Work out the finished part from the listing and answer in its coordinate system (mm). A direction names the side the tool comes from. Coordinates: 2 decimals unless noted, no trailing zeros. Loops run counter-clockwise (first coordinate to the right, second up) from the corner with the lowest first, then second, coordinate; pieces in that order, holes last. Notation, with made-up numbers: (-26.75, 59.25) -> (23.25, 59.25) arc R24 ccw to (23.25, 92.25) -> close; hole circle Ø5 at (1.5, -27). An arc over 180 degrees is marked (long way). Use a Markdown table: item, result.
from build123d import *

# Parameters (mm, degrees)
CYLINDER004_R     = 2.5
CYLINDER004_DEPTH = 16.6
CYLINDER005_R     = 1.5
CYLINDER005_DEPTH = 9
CYLINDER008_R     = 1.5
CYLINDER008_DEPTH = 9
CYLINDER007_R     = 4.8
CYLINDER007_DEPTH = 7.3
CHAMFER003_SIZE   = 0.2
CYLINDER002_R     = 9
CYLINDER002_DEPTH = 0.7
CHAMFER_SIZE      = 0.2
CYLINDER003_R     = 9
CYLINDER003_DEPTH = 0.7
CHAMFER001_SIZE   = 0.2
CYLINDER_R        = 0.6
CYLINDER_DEPTH    = 7.6
ARRAY_COUNT       = 20
CYLINDER001_R     = 6.7
CYLINDER001_DEPTH = 7.6


with BuildPart() as cilindro004:
    # Cylinder004 → Cylinder004 (new body)
    with BuildSketch(Plane.XY):
        Circle(CYLINDER004_R)
    extrude(amount=CYLINDER004_DEPTH)


with BuildPart() as cilindro005:
    # Cylinder005 → Cylinder005 (new body)
    with BuildSketch(Plane(origin=(1, 0, 3.5), x_dir=(0, 0, -1), z_dir=(1, 0, 0))):
        Circle(CYLINDER005_R)
    extrude(amount=CYLINDER005_DEPTH)


with BuildPart() as fusion001:
    # Cylinder008 → Cylinder008 (new body)
    with BuildSketch(Plane(origin=(0, -1, 3.5), x_dir=(0, 0, -1), z_dir=(0, -1, 0))):
        Circle(CYLINDER008_R)
    extrude(amount=CYLINDER008_DEPTH)

    # Fusion001: union Cilindro005
    add(cilindro005.part)


with BuildPart() as cut001:
    # Cylinder007 → Cylinder007 (new body)
    with BuildSketch(Plane.XY):
        Circle(CYLINDER007_R)
    extrude(amount=CYLINDER007_DEPTH)

    # Chamfer003
    chamfer003_edges = [cut001.edges().sort_by_distance(p)[0] for p in [
        (-4.8, 0, 7.3),
    ]]
    chamfer(chamfer003_edges, length=CHAMFER003_SIZE)

    # Cut001: cut Fusion001
    add(fusion001.part, mode=Mode.SUBTRACT)


with BuildPart() as cut001_1:
    # Cut001 placement: moved
    add(cut001.part.moved(Location((0, 0, 9))))


with BuildPart() as chamfer_body:
    # Cylinder002 → Cylinder002 (new body)
    with BuildSketch(Plane.XY):
        Circle(CYLINDER002_R)
    extrude(amount=CYLINDER002_DEPTH)

    # Chamfer
    chamfer_edges = [chamfer_body.edges().sort_by_distance(p)[0] for p in [
        (-9, 0, 0.7),
    ]]
    chamfer(chamfer_edges, length=CHAMFER_SIZE)


with BuildPart() as chamfer001:
    # Cylinder003 → Cylinder003 (new body)
    with BuildSketch(Plane.XY.offset(8.3)):
        Circle(CYLINDER003_R)
    extrude(amount=CYLINDER003_DEPTH)

    # Chamfer001
    chamfer001_edges = [chamfer001.edges().sort_by_distance(p)[0] for p in [
        (-9, 0, 8.3),
    ]]
    chamfer(chamfer001_edges, length=CHAMFER001_SIZE)


with BuildPart() as array:
    # Cylinder → Cylinder (new body)
    with BuildSketch(Plane(origin=(6.7, 0, 0), x_dir=(1, 0, 0), z_dir=(0, 0, 1))):
        Circle(CYLINDER_R)
    extrude(amount=CYLINDER_DEPTH)

    # Array: Array ×20 about axis
    array_axis = Axis((0, 0, 0), (0, 0, 1))


with BuildPart() as array_1:
    add(array.part)
    for i in range(1, ARRAY_COUNT):
        add(array.part.rotate(array_axis, i * 360 / ARRAY_COUNT))


with BuildPart() as obj1:
    # Cylinder001 → Cylinder001 (new body)
    with BuildSketch(Plane.XY):
        Circle(CYLINDER001_R)
    extrude(amount=CYLINDER001_DEPTH)

    # Cut: cut Array
    add(array_1.part, mode=Mode.SUBTRACT)


with BuildPart() as obj1_1:
    # Cut placement: moved
    add(obj1.part.moved(Location((0, 0, 0.7))))

    # Fusion: union Chamfer body, Chamfer001
    add(chamfer_body.part)
    add(chamfer001.part)

    # Fusion002: union Cut001
    add(cut001_1.part)

    # Cut002: cut Cilindro004
    add(cilindro004.part, mode=Mode.SUBTRACT)


solid = obj1_1.part
Q1. For faces 4 (the cylindrical face through (5.967, -3.047, 4.447)), 5 (the cylindrical face through (-6.62, -1.04, 4.45)), 6 (the cylindrical face through (-1.04, 6.62, 4.45)), 7 (the cylindrical face through (-5.806, 1.873, 4.447)), determine the directions among +Z, -Z, +X, -X, +Y, -Y from which every point of the face is accessible in a straight line to the end or side of a thin tool.
Solved:
| item | result |
|---|---|
| face 4 | +X, -Y |
| face 5 | -X, -Y |
| face 6 | -X, +Y |
| face 7 | none |
Q2. Section D-D on z = 9.25 is taken. Determine the outline of the cut face in (x, y), and give its area (3 significant figures).
Solved:
| item | result |
|---|---|
| outline | circle Ø9.6 at (0, 0); hole circle Ø5 at (0, 0) |
| area | 52.7 mm² |
Q3. Given pin 1 Ø4.5 at (x, y) = (0, 0) entering from +Z; pin 2 Ø3 at (x, z) = (-2, 8) entering from +Y; pin 3 Ø2 at (x, z) = (5, 10.5) entering from +Y; pin 4 Ø5 at (x, z) = (0, 12.5) entering from +Y, each flat-ended and moving along its own axis, determine where each tip first touches the part or whether it passes through.
Solved:
| item | result |
|---|---|
| pin 1 | through |
| pin 2 | y = 8.98 |
| pin 3 | y = 2.65 |
| pin 4 | y = 4.8 |
Q4. Section C-C on z = 12.5 is taken. Determine the outline of the cut face in (x, y).
Solved:
| item | result |
|---|---|
| outline | (-1.5, -4.56) -> (-1.5, -2) arc R2.5 cw (long way) to (2, 1.5) -> (4.56, 1.5) arc R4.8 ccw (long way) to start; (1.5, -4.56) arc R4.8 ccw to (4.56, -1.5) -> (2, -1.5) arc R2.5 cw to (1.5, -2) -> close |
Q5. Determine the mould class of faces 1 (the cylindrical face through (5.97, 3.04, 4.45)), 2 (the cylindrical face through (-1.054, -6.617, 4.447)), 3 (the cylindrical face through (-1.464, -3.382, 12.825)) for opening direction X: pulls with the +X half, pulls with the -X half, needs draft (parallel to the pull), parting line crosses it, or undercut.
Solved:
| item | result |
|---|---|
| face 1 | pulls with the +X half |
| face 2 | pulls with the -X half |
| face 3 | undercut |
Q6. Section A-A on x = 0 is taken. State how many separate pieces and enclosed holes the cut face has, and give its area (3 significant figures).
Solved:
| item | result |
|---|---|
| separate pieces | 3 |
| enclosed holes | 0 |
| area | 99.5 mm² |
Q7. Consider line 1 (Z direction, x = 7.5, y = 1.25); line 2 (Z direction, x = 3.4, y = 0); line 3 (X direction, y = -4.1, z = 12.5). Determine where each line is inside the solid, lowest interval first. Write a range as [from, to].
Solved:
| item | result |
|---|---|
| line 1 | [0, 0.7], [8.3, 9] |
| line 2 | [0, 11], [14, 16.3] |
| line 3 | [-2.5, -1.5], [1.5, 2.5] |
